from build123d import *

# Parameters (mm, degrees)
BOSS_EXTRUDE1_DEPTH  = 3.175
SKETCH3_R            = 5
CUT_EXTRUDE1_DEPTH   = 150.117288149
M3_CLEARANCE_HOLE1_D = 3.4
CUT_EXTRUDE2_DEPTH   = 150.117288149


with BuildPart() as part:
    # Sketch1 → Boss-Extrude1 (new body)
    with BuildSketch(Plane(origin=(0, 0, 0), x_dir=(1, 0, 0), z_dir=(0, 1, 0))):
        Polygon((-25, 0), (-25, 45.75), (25, 45.75), (25, 0), (31.35, 0), (31.35, -100), (25, -100), (25, -145.75), (-25, -145.75), (-25, -100), align=None)
    extrude(amount=BOSS_EXTRUDE1_DEPTH)

    # Sketch3 → Cut-Extrude1 (cut, through all)
    with BuildSketch(Plane(origin=(0, 3.175, 0), x_dir=(1, 0, 0), z_dir=(0, 1, 0))):
        with Locations(Location((0, -83.075, 0), (0, 0, 270))):
            Circle(SKETCH3_R)
    extrude(amount=-CUT_EXTRUDE1_DEPTH, mode=Mode.SUBTRACT)

    # M3 Clearance Hole1 (through all)
    with Locations(Plane(origin=(0, 3.175, 0), x_dir=(1, 0, 0), z_dir=(0, 1, 0))):
        with Locations((15.5, -98.575), (-15.5, -98.575), (-15.5, -67.575), (15.5, -67.575)):
            Hole(M3_CLEARANCE_HOLE1_D / 2)

    # Sketch6 → Cut-Extrude2 (cut, through all)
    with BuildSketch(Plane.XZ):
        with BuildLine():
            Line((17.2, 103.575), (17.2, 93.575))
            ThreePointArc((17.2, 93.575), (15.5, 91.875), (13.8, 93.575))
            Line((13.8, 93.575), (13.8, 103.575))
            ThreePointArc((13.8, 103.575), (15.5, 105.275), (17.2, 103.575))
        make_face()
        with BuildLine():
            Line((-13.8, 103.575), (-13.8, 93.575))
            ThreePointArc((-13.8, 93.575), (-15.5, 91.875), (-17.2, 93.575))
            Line((-17.2, 93.575), (-17.2, 103.575))
            ThreePointArc((-17.2, 103.575), (-15.5, 105.275), (-13.8, 103.575))
        make_face()
        with BuildLine():
            Line((17.2, 62.575), (17.2, 72.575))
            ThreePointArc((17.2, 72.575), (15.5, 74.275), (13.8, 72.575))
            Line((13.8, 72.575), (13.8, 62.575))
            ThreePointArc((13.8, 62.575), (15.5, 60.875), (17.2, 62.575))
        make_face()
        with BuildLine():
            Line((-13.8, 62.575), (-13.8, 72.575))
            ThreePointArc((-13.8, 72.575), (-15.5, 74.275), (-17.2, 72.575))
            Line((-17.2, 72.575), (-17.2, 62.575))
            ThreePointArc((-17.2, 62.575), (-15.5, 60.875), (-13.8, 62.575))
        make_face()
    extrude(amount=-CUT_EXTRUDE2_DEPTH, mode=Mode.SUBTRACT)


solid = part.part
Part model, mm, in its own coordinate system. A direction names the side the tool comes from. Coordinates: 2 decimals unless noted, no trailing zeros. Order: outer loops, then holes, each group sorted by start corner. A loop starts at its lowest first (then second) coordinate and runs counter-clockwise, first axis right, second up.
(1) Slice it at B-B, the plane x = 15.5. Write the cut outline in (y, z) (3 decimals).
Check sheet entries:
outline: (0, -45.75) - (3.175, -45.75) - (3.175, 60.875) - (0, 60.875) - close; (0, 74.275) - (3.175, 74.275) - (3.175, 91.875) - (0, 91.875) - close; (0, 105.275) - (3.175, 105.275) - (3.175, 145.75) - (0, 145.75) - close
(2) Tool access for faces 4 (the face through (31.35, 2, 49)), 5 (the face through (13.8, 2, 68)), 6 (the face through (25, 2, 123)), 7 (the face through (28, 2, 0)): list every direction of +Z, -Z, +X, -X, +Y, -Y with a clear straight run to the whole face (end or side of a thin tool).
Check sheet entries:
face 4: +Z, -Z, +X, +Y, -Y
face 5: +Y, -Y
face 6: +Z, +X, +Y, -Y
face 7: -Z, +X, +Y, -Y
(3) Pull direction Z, two halves, no side cores. Call faces 1 (the face through (0, 2, 145.75)), 2 (the face through (4, 0, 49)), 3 (the face through (15.463, 1.565, 60.875)): pulls with the +Z half, pulls with the -Z half, needs draft (parallel to the pull), parting line crosses it, or undercut.
Check sheet entries:
face 1: pulls with the +Z half
face 2: needs draft
face 3: undercut
(4) Slice it at A-A, the plane x = 0. Write the cut outline in (y, z) (3 decimals), and give its area (3 significant figures).
Check sheet entries:
outline: (0, -45.75) - (3.175, -45.75) - (3.175, 78.075) - (0, 78.075) - close; (0, 88.075) - (3.175, 88.075) - (3.175, 145.75) - (0, 145.75) - close
area: 576 mm2
(5) Slice it at D-D, the plane z = -2. Write the cut outline in (x, y) (3 decimals).
Check sheet entries:
outline: (-25, 0) - (25, 0) - (25, 3.175) - (-25, 3.175) - close
(6) Probe L1, parallel to X at y = 2.3, z = 64.5; L2, parallel to X at y = 2.45, z = 130.5; L3, parallel to X at y = 2.75, z = 86. List the from-to ranges inside material, lowest first.
Check sheet entries:
L1: x = -25 to -17.2, -13.8 to 13.8, 17.2 to 31.35
L2: x = -25 to 25
L3: x = -25 to -4.06, 4.06 to 31.35
(7) Slice it at C-C, the plane y = 2.3. Write the cut outline in (x, z) (3 decimals).
Check sheet entries:
outline: (-25, -45.75) - (25, -45.75) - (25, 0) - (31.35, 0) - (31.35, 100) - (25, 100) - (25, 145.75) - (-25, 145.75) - close; hole (-17.2, 62.575) arc R1.7 ccw to (-13.8, 62.575) - (-13.8, 72.575) arc R1.7 ccw to (-17.2, 72.575) - close; hole (-17.2, 93.575) arc R1.7 ccw to (-13.8, 93.575) - (-13.8, 103.575) arc R1.7 ccw to (-17.2, 103.575) - close; hole circle Ø10 at (0, 83.075); hole (13.8, 62.575) arc R1.7 ccw to (17.2, 62.575) - (17.2, 72.575) arc R1.7 ccw to (13.8, 72.575) - close; hole (13.8, 93.575) arc R1.7 ccw to (17.2, 93.575) - (17.2, 103.575) arc R1.7 ccw to (13.8, 103.575) - close
(8) Pin check, flat tips, straight feed: pin 1 Ø1.6 at (y, z) = (1.5, 123.5) entering from +X; pin 2 Ø9 at (x, z) = (0, 83.075) entering from -Y; pin 3 Ø1 at (x, y) = (29, 1.5) entering from -Z. Stop position of each tip, or through.
Check sheet entries:
pin 1: stops at x = 25
pin 2: passes through
pin 3: stops at z = 0
